from build123d import *

# Parameters (mm, degrees)
CONG_1_R                = 0.5
ESQUISSE2_R             = 6
ENL_V_MAT_EXTRU_1_DEPTH = 20.410049083
CONG_2_R                = 0.5


with BuildPart() as part:
    # Esquisse1 → Base-Révolution (revolve)
    with BuildSketch(Plane.XY, mode=Mode.PRIVATE) as base_r_volution_sk:
        with BuildLine():
            Line((0, 0), (0, 7.341687605))
            ThreePointArc((0, 7.341687605), (0.5, 9), (0, 10.658312395))
            Line((0, 10.658312395), (0, 13.5))
            Line((0, 13.5), (3.5, 13.5))
            Line((3.5, 13.5), (3.5, 0))
            Line((3.5, 0), (0, 0))
        make_face()
    revolve(base_r_volution_sk.sketch.rotate(Axis((-2.5, 0, 0), (1, 0, 0)), 270), axis=Axis((-2.5, 0, 0), (1, 0, 0)))

    # Congé1
    cong_1_edges = [part.edges().sort_by_distance(p)[0] for p in [
        (3.5, 0, 13.5),
    ]]
    fillet(cong_1_edges, radius=CONG_1_R)

    # Esquisse2 → Enlèv. mat.-Extru.1 (cut, through all)
    with BuildSketch(Plane(origin=(3.5, 0, 0), x_dir=(0, 0, -1), z_dir=(1, 0, 0))):
        Circle(ESQUISSE2_R)
    extrude(amount=-ENL_V_MAT_EXTRU_1_DEPTH, mode=Mode.SUBTRACT)

    # Congé2
    cong_2_edges = [part.edges().sort_by_distance(p)[0] for p in [
        (3.5, 0, 6),
    ]]
    fillet(cong_2_edges, radius=CONG_2_R)


solid = part.part
Work out the finished part from the listing and answer in its coordinate system (mm). Round coordinates to 2 decimals unless told otherwise and drop trailing zeros. Write each loop counter-clockwise with the first axis right and the second up, starting at its lowest first coordinate (ties: lowest second). Pieces come first, ordered by that corner, then holes. Notation, with made-up numbers: (-3.5, 54.25) - (51.5, 54.25) arc R16 ccw to (51.5, 76.25) - close; hole circle Ø3 at (88, 49.25). An arc over 180 degrees is marked (long way). Answer in a Markdown table with one row per item. Add a question column.
1. A cutting plane is placed at A-A, the plane y = 0. Determine the outline of the cut face in (x, z), and give its area (3 significant figures).
2. The mould has two halves that part along Y. Classify faces 1 (the cylindrical face through (2, 0, 6)), 2 (the cylindrical face through (1.52, -13.18, 2.93)), 3 (the flat face through (0, -3.9, -10.1)): +Y half, -Y half, draft (parallel to the pull), parting line (faces both ways), or undercut.
3. A cutting plane is placed at C-C, the plane x = 2.35. Determine the outline of the cut face in (y, z).
4. Given pin 1 (2 mm diameter, centred on x = 2, y = -7.5, fed in from +Z), flat-ended and moving along its own axis, determine where the tip first touches the part or whether it passes through.
5. Find the intervals of material crossed by line 1 along Y through (x, z) = (1.05, 0); line 2 along X through (y, z) = (-8.5, -3); line 3 along Z through (x, y) = (1.05, 2.5), in increasing order. Write a range as from..to.
Worked out:
| question | item | result |
|---|---|---|
| 1 | outline | (0, -13.5) - (3, -13.5) arc R0.5 ccw to (3.5, -13) - (3.5, -6.5) arc R0.5 ccw to (3, -6) - (0, -6) - (0, -7.34) arc R3 cw to (0, -10.66) - close; (0, 6) - (3, 6) arc R0.5 ccw to (3.5, 6.5) - (3.5, 13) arc R0.5 ccw to (3, 13.5) - (0, 13.5) - (0, 10.66) arc R3 cw to (0, 7.34) - close |
| 1 | area | 50.0 mm^2 |
| 2 | face 1 | undercut |
| 2 | face 2 | parting line |
| 2 | face 3 | draft |
| 3 | outline | circle Ø27 at (0, 0); hole circle Ø12 at (0, 0) |
| 4 | pin 1 | z = 11.83 |
| 5 | line 1 | -13.5..-6, 6..13.5 |
| 5 | line 2 | 0.5..3.5 |
| 5 | line 3 | -13.27..-5.45, 5.45..13.27 |
